Verification items for the finished model (mm, model axes). A direction names the side the tool comes from. Coordinates: 2 decimals unless noted, no trailing zeros. Write each loop counter-clockwise with the first axis right and the second up, starting at its lowest first coordinate (ties: lowest second). Pieces come first, ordered by that corner, then holes. Notation, with made-up numbers: (78.5, 55.25) - (122.5, 55.25) arc R24 cw to (122.5, 76.25) - close; hole circle Ø11 at (69, 70). An arc over 180 degrees is marked (long way). Use CSV: the item, a comma, the result in double quotes. Start each with the question number.
```python
from build123d import *

# Parameters (mm, degrees)
BOSS_EXTRUDE1_DEPTH = 25
CUT_EXTRUDE1_REACH  = 99.811
SKETCH6_R           = 7.89
FILLET1_R           = 12.5
FILLET2_R           = 12.5
SKETCH7_R           = 12.5
SKETCH7_R_2         = 6.79
BOSS_EXTRUDE2_DEPTH = 3
SKETCH8_R           = 7.89
CUT_EXTRUDE2_DEPTH  = 5
CUT_EXTRUDE3_REACH  = 99.93
SKETCH9_R           = 1.7


with BuildPart() as part:
    # Sketch2 → Boss-Extrude1 (new body)
    with BuildSketch(Plane.XY):
        with BuildLine():
            Line((0, 53), (-25, 53))
            Line((-25, 53), (-25, 50))
            Line((-25, 50), (0, 50))
            ThreePointArc((0, 50), (35.509268781, 35.200736223), (49.998096153, -0.436326775))
            Line((49.998096153, -0.436326775), (49.779932766, -25.435374852))
            Line((49.779932766, -25.435374852), (52.779818535, -25.461554458))
            Line((52.779818535, -25.461554458), (52.997981922, -0.462506381))
            ThreePointArc((52.997981922, -0.462506381), (37.639824908, 37.312780396), (0, 53))
        make_face()
    extrude(amount=BOSS_EXTRUDE1_DEPTH)

    # Sketch6 → Cut-Extrude1 (cut, up to next)
    with BuildSketch(Plane(origin=(52.997981922, -0.462506381, 0), x_dir=(0, 0, -1), z_dir=(0.9999619230641714, -0.00872653549837746, 0)), mode=Mode.PRIVATE) as cut_extrude1_sk1:
        with Locations(Location((-12.5, -12.5, 0), (0, 0, 90))):
            Circle(SKETCH6_R)
    cut_extrude1_tool1 = extrude(cut_extrude1_sk1.sketch, amount=-CUT_EXTRUDE1_REACH, mode=Mode.PRIVATE) & part.part
    add(cut_extrude1_tool1.solids().sort_by_distance((52.8889, -12.96203, 12.5))[0], mode=Mode.SUBTRACT)

    # Fillet1
    fillet1_edges = [part.edges().sort_by_distance(p)[0] for p in [
        (51.27987565, -25.448464655, 0),
        (51.27987565, -25.448464655, 25),
    ]]
    fillet(fillet1_edges, radius=FILLET1_R - 0.0001)  # a hair under: the kernel refuses the full size

    # Fillet2
    fillet2_edges = [part.edges().sort_by_distance(p)[0] for p in [
        (-25, 51.5, 25),
        (-25, 51.5, 0),
    ]]
    fillet(fillet2_edges, radius=FILLET2_R - 0.0001)  # a hair under: the kernel refuses the full size

    # Sketch7 → Boss-Extrude2 (add)
    with BuildSketch(Plane(origin=(49.998096153, -0.436326775, 0), x_dir=(0, 0, 1), z_dir=(-0.9999619230641714, 0.008726535498377049, 0))):
        with Locations(Location((12.5, -12.5, 0), (0, 0, 270))):
            Circle(SKETCH7_R)
        with Locations(Location((12.5, -12.5, 0), (0, 0, 270))):
            Circle(SKETCH7_R_2, mode=Mode.SUBTRACT)
    extrude(amount=BOSS_EXTRUDE2_DEPTH)

    # Sketch8 → Cut-Extrude2 (cut)
    with BuildSketch(Plane(origin=(52.997981922, -0.462506381, 0), x_dir=(0, 0, -1), z_dir=(0.9999619230641714, -0.00872653549837732, 0))):
        with Locations(Location((-12.5, -12.5, 0), (0, 0, 90))):
            Circle(SKETCH8_R)
    extrude(amount=-CUT_EXTRUDE2_DEPTH, mode=Mode.SUBTRACT)

    # Sketch9 → Cut-Extrude3 (cut, up to next)
    with BuildSketch(Plane(origin=(0, 53, 0), x_dir=(1, 0, 0), z_dir=(0, 1, 0)), mode=Mode.PRIVATE) as cut_extrude3_sk1:
        with Locations(Location((-12.5, -12.5, 0), (0, 0, 270))):
            Circle(SKETCH9_R)
    cut_extrude3_tool1 = extrude(cut_extrude3_sk1.sketch, amount=-CUT_EXTRUDE3_REACH, mode=Mode.PRIVATE) & part.part
    add(cut_extrude3_tool1.solids().sort_by_distance((-12.5, 53, 12.5))[0], mode=Mode.SUBTRACT)


solid = part.part
```
Q1. Gauge pin test, flat ends, axial feed: pin 1 (12 mm diameter, centred on x = 36.5, z = 19, fed in from -Y); pin 2 (1 mm diameter, centred on y = 30.5, z = 5.5, fed in from -X); pin 3 (8 mm diameter, centred on y = 44, z = 6, fed in from +X). Record the tip position at first contact, or that the pin passes through.
Q2. Scan lines: line 1 along Y through (x, z) = (-16.5, 23.5); line 2 along Z through (x, y) = (-12, 51); line 3 along X through (y, z) = (8.5, 19). Record each from-to range of solid material in increasing order. Write a range as from..to.
Q3. Release check for a two-part mould opening along X. For faces 3 (the cylindrical face through (35.12, 35.59, 12.32)), 4 (the cylindrical face through (-11.99, 51.52, 14.12)) record: released by +X, released by -X, zero draft, split by the parting line, or undercut.
Q4. Tool access check on faces 1 (the flat face through (-10, 50, 12)), 2 (the cylindrical face through (-21.436, 51.479, 21.241)). Record the directions out of +Z, -Z, +X, -X, +Y, -Y that give a thin tool (end or side, any length) a straight path to the whole face; none if there is none.
Q5. Cross-section at A-A (z = 17.25). Record the cut outline in (x, y).
Q6. Cross-section at C-C (y = 38.5). Record the cut outline in (x, z).
Q7. Cross-section at B-B (x = -6.5). Record the cut outline in (y, z).
Reply:
1,pin 1,"y = 26.34"
1,pin 2,"x = 39.23"
1,pin 3,"x = 34.77"
2,line 1,"50..53"
2,line 2,"0..10.88, 14.12..25"
2,line 3,"49.27..52.31"
3,face 3,"released by -X"
3,face 4,"undercut"
4,face 1,"+Z, -Z, -X, -Y"
4,face 2,"+Z, -X, +Y, -Y"
5,outline,"(-24.06, 50) - (0, 50) arc R50 cw to (50, -0.44) - (49.99, -1.37) - (46.99, -1.35) - (46.93, -8.06) - (47.93, -8.07) - (47.94, -6.62) - (52.94, -6.66) - (53, -0.46) arc R53 ccw to (0, 53) - (-24.06, 53) - close; (46.79, -24.47) - (52.79, -24.52) - (52.83, -19.26) - (47.83, -19.22) - (47.85, -17.77) - (46.85, -17.76) - close"
6,outline,"(31.9, 0) - (36.42, 0) - (36.42, 25) - (31.9, 25) - close"
7,outline,"(50, 0) - (53, 0) - (53, 25) - (50, 25) - close"
